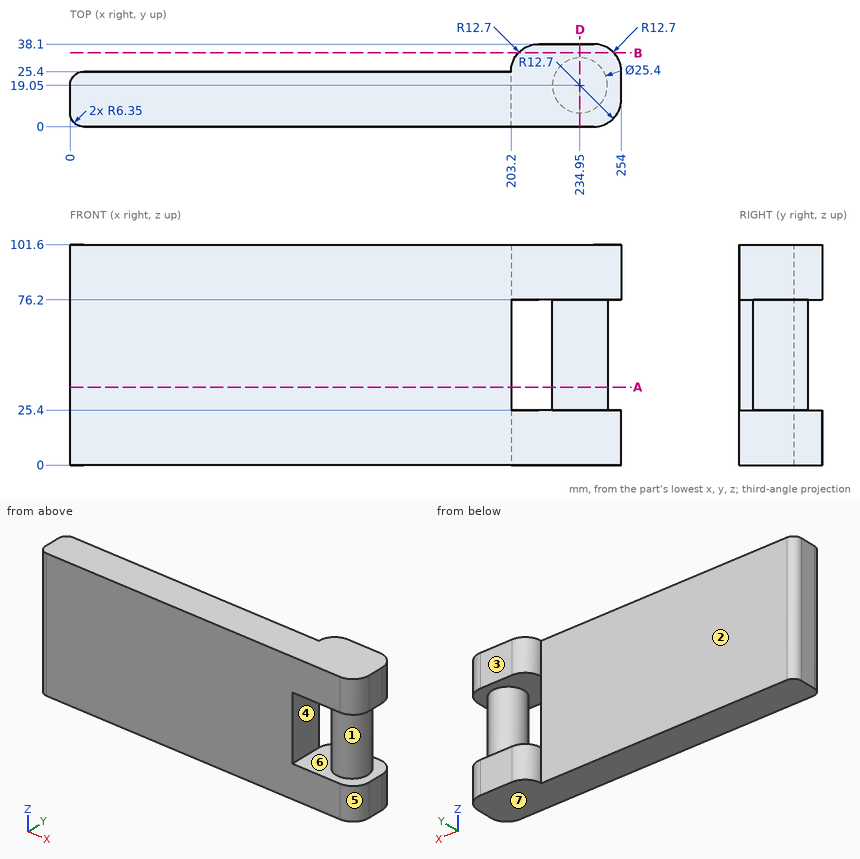
Here's the drawing with two shaded views (mm, measured from the low corner). I have some questions. A direction names the side the tool comes from. Round coordinates to 2 decimals unless told otherwise and drop trailing zeros. Order: outer loops, then holes, each group sorted by start corner. A loop starts at its lowest first (then second) coordinate and runs counter-clockwise, first axis right, second up. Notation, with made-up numbers: (77, -34) -> (109, -34) arc R25 cw to (109, -9) -> close; hole circle Ø11 at (-25, 69). An arc over 180 degrees is marked (long way). Use a Markdown table: item, result. Add a question column.
(1) Suppose I cut it at A-A, the plane z = 36. Please give me the cut outline in (x, y), and give its area (3 significant figures).
(2) I need wall thicknesses on line 1 along Z through (x, y) = (210, 9.5); line 2 along Y through (x, z) = (72, 69); line 3 along X through (y, z) = (19.5, 31.5) (1 decimal). Which ranges of each line are inside material? Lowest first, please.
(3) Suppose I cut it at D-D, the plane x = 234.95. Please give me the cut outline in (y, z).
(4) Suppose I cut it at B-B, the plane y = 34. Please give me the cut outline in (x, z) (1 decimal).
(5) For the marked faces 1, 2 and 3, which set-ups out of +Z, -Z, +X, -X, +Y, -Y let a thin tool reach every point of the face, with its end or its side?
(6) For pin 1 Ø4 at (x, z) = (168.5, 25.5) entering from -Y; pin 2 Ø1 at (x, z) = (183, 13.5) entering from +Y, each with a flat end and sliding along its axis, tell me the tip position at first contact or that it passes through.
(7) If we mould it in two halves opening along X, with no side actions, what happens to the marked faces 4, 5, 6 and 7? For each: released by +X, released by -X, zero draft, split by the parting line, or undercut.
Verdict:
| question | item | result |
|---|---|---|
| 1 | outline | (0, 6.35) arc R6.35 ccw to (6.35, 0) -> (203.2, 0) -> (203.2, 25.4) -> (6.35, 25.4) arc R6.35 ccw to (0, 19.05) -> close; circle Ø25.4 at (234.95, 19.05) |
| 1 | area | 5,650 mm2 |
| 2 | line 1 | 0 to 25.4, 76.2 to 101.6 |
| 2 | line 2 | 0 to 25.4 |
| 2 | line 3 | 0 to 203.2, 222.3 to 247.6 |
| 3 | outline | (0, 0) -> (38.1, 0) -> (38.1, 25.4) -> (31.75, 25.4) -> (31.75, 76.2) -> (38.1, 76.2) -> (38.1, 101.6) -> (0, 101.6) -> (0, 76.2) -> (6.35, 76.2) -> (6.35, 25.4) -> (0, 25.4) -> close |
| 4 | outline | (206.6, 0) -> (250.6, 0) -> (250.6, 25.4) -> (206.6, 25.4) -> close; (206.6, 76.2) -> (250.6, 76.2) -> (250.6, 101.6) -> (206.6, 101.6) -> close |
| 5 | face 1 | none |
| 5 | face 2 | +Z, -Z, -X, +Y |
| 5 | face 3 | +Z, -Z, +X, -X, +Y |
| 6 | pin 1 | y = 0 |
| 6 | pin 2 | y = 25.4 |
| 7 | face 4 | undercut |
| 7 | face 5 | released by +X |
| 7 | face 6 | undercut |
| 7 | face 7 | zero draft |
